```python
from build123d import *

# Parameters (mm, degrees)
BOSS_EXTRUDE1_DEPTH = 2.975
SKETCH2_R           = 2.175
SKETCH2_R_2         = 2.175000000000007
CUT_EXTRUDE1_DEPTH  = 12.7
SKETCH3_R           = 2.175000000000007
BOSS_EXTRUDE2_DEPTH = 3.7750000000000004


with BuildPart() as part:
    # Sketch1 → Boss-Extrude1 (new body)
    with BuildSketch(Plane(origin=(0, 0, 0), x_dir=(1, 0, 0), z_dir=(0, 1, 0))):
        with BuildLine():
            Line((-23.171929824561392, 5.625877192982455), (56.3300701754386, 5.625877192982454))
            ThreePointArc((56.3300701754386, 5.625877192982454), (62.6800701754386, -0.7241228070175446), (56.3300701754386, -7.074122807017544))
            Line((56.3300701754386, -7.074122807017544), (-23.171929824561392, -7.074122807017544))
            ThreePointArc((-23.171929824561392, -7.074122807017544), (-29.52192982456139, -0.7241228070175436), (-23.171929824561392, 5.625877192982455))
        make_face()
    extrude(amount=BOSS_EXTRUDE1_DEPTH)

    # Sketch2 → Cut-Extrude1 (cut)
    with BuildSketch(Plane(origin=(0, 2.975, 0), x_dir=(1, 0, 0), z_dir=(0, 1, 0))):
        with Locations(Location((-23.171929824561392, -0.7241228070175446, 0), (0, 0, 270))):
            Circle(SKETCH2_R)
        with Locations(Location((56.3300701754386, -0.7241228070175446, 0), (0, 0, 270))):
            Circle(SKETCH2_R_2)
    extrude(amount=-CUT_EXTRUDE1_DEPTH, mode=Mode.SUBTRACT)

    # Sketch3 → Boss-Extrude2 (add)
    with BuildSketch(Plane(origin=(0, 2.975, 0), x_dir=(1, 0, 0), z_dir=(0, 1, 0))):
        with BuildLine():
            ThreePointArc((56.3300701754386, 5.625877192982454), (62.6800701754386, -0.7241228070175451), (56.3300701754386, -7.074122807017544))
            ThreePointArc((56.3300701754386, -7.074122807017544), (49.9800701754386, -0.7241228070175443), (56.3300701754386, 5.625877192982454))
        make_face()
        with Locations(Location((56.3300701754386, -0.7241228070175446, 0), (0, 0, 270))):
            Circle(SKETCH3_R, mode=Mode.SUBTRACT)
    extrude(amount=BOSS_EXTRUDE2_DEPTH)


solid = part.part
```
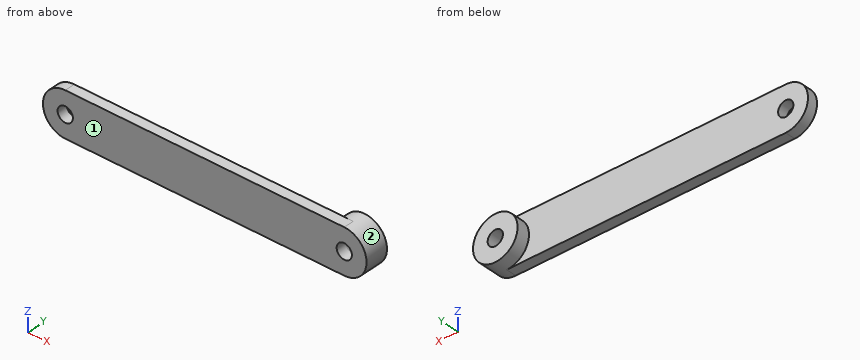
Can you work these out from the model? Positions are in its coordinate system, mm. Face numbers are marked on the shaded views. A direction names the side the tool comes from. Give positions to 0.01 mm unless a question says otherwise; leave off trailing zeros. Loops run counter-clockwise (first coordinate to the right, second up) from the corner with the lowest first, then second, coordinate; pieces in that order, holes last. Notation, with made-up numbers: M 78.5,49 L 123.5,49 A13 ccw 123.5,59 Z; hole C -12,2.5 d8. An arc over 180 degrees is marked long. Use one line per item in the form item = value. Start each with the question number.
(1) Please list where these lines run through material, in increasing order: line 1 (X direction, y = 5, z = 0.5); line 2 (X direction, y = 1.25, z = 2.25); line 3 (Y direction, x = -6, z = 3.25) (3 decimals).
(2) I want a section at C-C, the plane y = 5.5. Write out the boundary of the cut face in (x, z) (3 decimals), and give its area (3 significant figures).
(3) I want a section at D-D, the plane x = 36. Write out the boundary of the cut face in (y, z) (3 decimals).
(4) I want a section at A-A, the plane z = 0. State how many separate pieces and enclosed holes the cut face has, and give its area (3 significant figures).
(5) I'm going to push flat-ended pins straight in: P1, Ø3, axis at x = 43, z = -3, coming from the +Y side (3 decimals); P2, Ø4, axis at x = -23.17, z = 0.72, coming from the +Y side; P3, Ø1.5, axis at y = 2, z = 2.5, coming from the +X side. Where does each tip first touch, or does it pass through?
(6) On a 3-axis mill with a long thin cutter (end or side, diameter ignored), from which of +Z, -Z, +X, -X, +Y, -Y can I reach the whole of each face in a straight line? I mean the marked faces 1 and 2. Say none if no direction works.
(7) I want a section at B-B, the plane y = 0.75. Write out the boundary of the cut face in (x, z) (3 decimals).
Worked out:
q1.line_1 = 49.98 to 54.17, 58.49 to 62.68
q1.line_2 = -29.34 to -24.72, -21.62 to 54.78, 57.88 to 62.49
q1.line_3 = 0 to 2.975
q2.outline = C 56.33,0.724 d12.7; hole C 56.33,0.724 d4.35
q2.area = 112 mm²
q3.outline = M 0,-5.626 L 2.975,-5.626 L 2.975,7.074 L 0,7.074 Z
q4.separate_pieces = 3
q4.enclosed_holes = 0
q4.area = 282 mm²
q5.P1 = 2.975
q5.P2 = through
q5.P3 = 62.6
q6.face_1 = +Z, -Z, +X, -X, -Y
q6.face_2 = +Y
q7.outline = M -23.172,-5.626 L 56.33,-5.626 A6.35 ccw 56.33,7.074 L -23.172,7.074 A6.35 ccw Z; hole C -23.172,0.724 d4.35; hole C 56.33,0.724 d4.35
